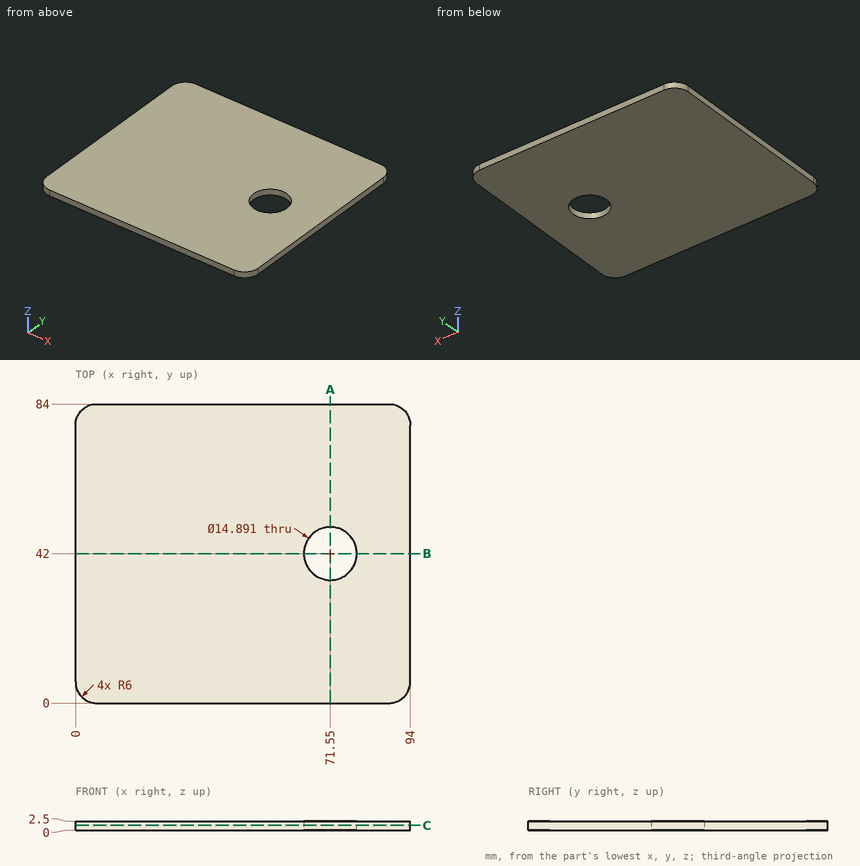
Print and shaded views of the part. All mm, measured from the part's lowest x, y and z. Coordinates: 2 decimals unless noted, no trailing zeros. Order: outer loops, then holes, each group sorted by start corner. A loop starts at its lowest first (then second) coordinate and runs counter-clockwise, first axis right, second up. Notation, with made-up numbers: (-32.75, -21.5) - (23.25, -21.5) arc R22 ccw to (23.25, -10.5) - close; hole circle Ø1 at (-6, -4.5). An arc over 180 degrees is marked (long way). Put each result on its own line as item: value.
1. Saw through at A-A (x = 71.55). Write the cut outline in (y, z).
Answer sheet:
outline: (0, 0) - (34.55, 0) - (34.55, 2.5) - (0, 2.5) - close; (49.45, 0) - (84, 0) - (84, 2.5) - (49.45, 2.5) - close
2. Saw through at C-C (z = 1.3). Write the cut outline in (x, y).
Answer sheet:
outline: (0, 6) arc R6 ccw to (6, 0) - (88, 0) arc R6 ccw to (94, 6) - (94, 78) arc R6 ccw to (88, 84) - (6, 84) arc R6 ccw to (0, 78) - close; hole circle Ø14.89 at (71.55, 42)
3. Saw through at B-B (y = 42). Write the cut outline in (x, z).
Answer sheet:
outline: (0, 0) - (64.1, 0) - (64.1, 2.5) - (0, 2.5) - close; (79, 0) - (94, 0) - (94, 2.5) - (79, 2.5) - close
4. Probe line 1 along Y through (x, z) = (71.55, 1.05); line 2 along X through (y, z) = (38, 0.45); line 3 along Y through (x, z) = (67.5, 2.15). List the from-to ranges inside material, lowest first. Write a range as [from, to].
Answer sheet:
line 1: y = [0, 34.55], [49.45, 84]
line 2: x = [0, 65.27], [77.83, 94]
line 3: y = [0, 35.75], [48.25, 84]
